from build123d import *

# Parameters (mm, degrees)
SKETCH014_R      = 3.55
EXTRUDE004_DEPTH = 4.7
POCKET_DEPTH     = 2
FILLET006_R      = 2


with BuildPart() as part:
    # Sketch014 → Extrude004 (new body)
    with BuildSketch(Plane.XY):
        with BuildLine():
            Line((-6.25, 21.219667), (-3.1, 21.219667))
            Line((-3.1, 21.219667), (-3.1, 11.042747))
            ThreePointArc((-3.1, 11.042747), (-2.514214, 9.628534), (-1.1, 9.042747))
            Line((-1.1, 9.042747), (1.1, 9.042747))
            ThreePointArc((1.1, 9.042747), (2.514214, 9.628534), (3.1, 11.042747))
            Line((3.1, 21.219667), (3.1, 11.042747))
            Line((3.1, 21.219667), (6.25, 21.219667))
            Line((6.25, 21.219667), (6.25, 7.219667))
            Line((6.25, 7.219667), (5.996507, -0.204713))
            ThreePointArc((-6, 0), (-0.102371, -5.999127), (5.996507, -0.204713))
            Line((-6.25, 7.219635), (-6, 0))
            Line((-6.25, 7.219635), (-6.25, 21.219667))
        make_face()
        Circle(SKETCH014_R, mode=Mode.SUBTRACT)
    extrude(amount=EXTRUDE004_DEPTH)

    # Sketch015 (on Face15 of Extrude004) → Pocket (cut)
    with BuildSketch(Plane.XY.offset(4.7)):
        with BuildLine():
            ThreePointArc((-2.825, 2.149855), (0, -3.55), (2.825, 2.149855))
            Line((2.825, 2.149855), (2.4, 9.919679))
            Line((-2.4, 9.919679), (2.4, 9.919679))
            Line((-2.825, 2.149855), (-2.4, 9.919679))
        make_face()
    extrude(amount=-POCKET_DEPTH, mode=Mode.SUBTRACT)

    # Fillet006
    fillet006_edges = [part.edges().sort_by_distance(p)[0] for p in [
        (6.25, 21.219667, 2.35),
        (-6.25, 21.219667, 2.35),
    ]]
    fillet(fillet006_edges, radius=FILLET006_R)


solid = part.part
The model under review builds one solid part; all positions refer to its coordinate system, in mm. A direction names the side the tool comes from. Coordinates: 2 decimals unless noted, no trailing zeros. Order: outer loops, then holes, each group sorted by start corner. A loop starts at its lowest first (then second) coordinate and runs counter-clockwise, first axis right, second up. Notation, with made-up numbers: (69, 41.25) -> (127, 41.25) arc R33 ccw to (127, 77.25) -> close; hole circle Ø5 at (40.5, -24). An arc over 180 degrees is marked (long way). Answer in a Markdown table with one row per item.
(1) Consider section B-B (y = 13.25). Write out the cut boundary in (x, z), plus the area to 3 significant figures.
Answers:
| item | result |
|---|---|
| outline | (-6.25, 0) -> (-3.1, 0) -> (-3.1, 4.7) -> (-6.25, 4.7) -> close; (3.1, 0) -> (6.25, 0) -> (6.25, 4.7) -> (3.1, 4.7) -> close |
| area | 29.6 mm² |
(2) Insertion check: pin 1 (4 mm diameter, centred on x = -1, y = 1, fed in from -Z); pin 2 (6 mm diameter, centred on x = 0.5, y = 5, fed in from +Z); pin 3 (1.8 mm diameter, centred on x = 0.5, z = 2, fed in from +Y); pin 4 (1.5 mm diameter, centred on y = 1.5, z = 4, fed in from +X). Each pin has a flat end and moves straight along its axis. Give the tip position at first contact, or say it passes through.
Answers:
| item | result |
|---|---|
| pin 1 | through |
| pin 2 | z = 4.7 |
| pin 3 | y = 9.07 |
| pin 4 | x = 6.08 |
(3) Machinability: for faces 5 (the flat face through (2.626, 5.794, 3.714)), 6 (the cylindrical face through (2.726, 9.878, 1.795)), 7 (the flat face through (-3, 8, 4.7)), which of the approach directions +Z, -Z, +X, -X, +Y, -Y give a long, thin tool a straight path to every point of the face, cutting with its end or side? Answer none if there is none.
Answers:
| item | result |
|---|---|
| face 5 | +Z |
| face 6 | +Z, -Z, +Y |
| face 7 | +Z, +X, -X, +Y, -Y |
(4) Wall thickness on line 1 along X through (y, z) = (12, 3.9); line 2 along Y through (x, z) = (0, 1.95); line 3 along X through (y, z) = (-3.25, 3.9): over which ranges is each line inside the solid? List them lowest first.
Answers:
| item | result |
|---|---|
| line 1 | -6.25 to -3.1, 3.1 to 6.25 |
| line 2 | -6 to -3.55, 3.55 to 9.04 |
| line 3 | -5.04 to -1.43, 1.43 to 5.04 |
(5) Consider section A-A (x = 0). Write out the cut boundary in (y, z), plus the area to 3 significant figures.
Answers:
| item | result |
|---|---|
| outline | (-6, 0) -> (-3.55, 0) -> (-3.55, 4.7) -> (-6, 4.7) -> close; (3.55, 0) -> (9.04, 0) -> (9.04, 2.7) -> (3.55, 2.7) -> close |
| area | 26.3 mm² |
(6) The part is to be moulded in two halves that separate along Y. For faces 1 (the flat face through (-4, 21.22, 2)), 2 (the flat face through (-2.626, 5.794, 3.714)), 3 (the cylindrical face through (-0.77, -3.466, 2.317)), 4 (the flat face through (6.25, 13, 2)), say which applies: +Y half, -Y half, draft (parallel to the pull), parting line (faces both ways), or undercut.
Answers:
| item | result |
|---|---|
| face 1 | +Y half |
| face 2 | undercut |
| face 3 | undercut |
| face 4 | draft |
(7) Consider section D-D (z = 1.05). Write out the cut boundary in (x, y).
Answers:
| item | result |
|---|---|
| outline | (-6.25, 7.22) -> (-6, 0) arc R6 ccw to (6, -0.2) -> (6.25, 7.22) -> (6.25, 19.22) arc R2 ccw to (4.25, 21.22) -> (3.1, 21.22) -> (3.1, 11.04) arc R2 cw to (1.1, 9.04) -> (-1.1, 9.04) arc R2 cw to (-3.1, 11.04) -> (-3.1, 21.22) -> (-4.25, 21.22) arc R2 ccw to (-6.25, 19.22) -> close; hole circle Ø7.1 at (0, 0) |
